The listing builds one solid part. Answer for the finished solid, in the listing's coordinates (mm). A direction names the side the tool comes from. Give positions to 0.01 mm unless a question says otherwise; leave off trailing zeros. One line per question, with ' | ' between items. Start each with the question number.
1. Given P1, Ø17, axis at x = -3.175, y = -38.1, coming from the -Z side; P2, Ø4, axis at x = 17.5, z = -65, coming from the +Y side; P3, Ø15.5, axis at y = 53, z = 56.5, coming from the +X side, each flat-ended and moving along its own axis, determine where each tip first touches the part or whether it passes through.
2. Find the intervals of material crossed by L1, parallel to Y at x = 2, z = 57; L2, parallel to Z at x = -2, y = -23; L3, parallel to X at y = 38.1, z = -165 (3 decimals), in increasing order. Write a range as from..to.
3. The mould has two halves that part along Y. Classify faces 1 (the face through (18, 14.288, 3)), 2 (the face through (22.225, 36, 3)), 3 (the face through (-4, 57.15, 3)): +Y half, -Y half, draft (parallel to the pull), parting line (faces both ways), or undercut.
4. For faces 4 (the face through (-4.415, -47.544, -165.633)), 5 (the face through (18, 28.575, 3)), 6 (the face through (0.31, -22.15, 94.41)), determine the directions among +Z, -Z, +X, -X, +Y, -Y from which every point of the face is accessible in a straight line to the end or side of a thin tool.
5. A cutting plane is placed at B-B (z = -156.5). State how many separate pieces and enclosed holes the cut face has, then the cut area to 3 significant figures.
```python
from build123d import *

# Parameters (mm, degrees)
F1_DEPTH = 203.2
F2_R     = 5.55625
F3_DEPTH = 44.451
F4_R     = 9.525
F5_DEPTH = 76.2


with BuildPart() as f1:
    # F0 (on Top) → F1 (new body, symmetric)
    with BuildSketch(Plane.XY):
        Polygon((14.2875, 57.15), (-22.225, 57.15), (-22.225, -57.15), (22.225, -57.15), (22.225, -42.8625), (14.2875, -42.8625), (14.2875, -28.575), (22.225, -28.575), (22.225, -14.2875), (14.2875, -14.2875), (14.2875, 0), (22.225, 0), (22.225, 14.2875), (14.2875, 14.2875), (14.2875, 28.575), (22.225, 28.575), (22.225, 42.8625), (14.2875, 42.8625), align=None)
    extrude(amount=F1_DEPTH, both=True)

    # F2 (on face) → F3 (cut, through all)
    with BuildSketch(Plane.YZ.offset(22.225)):
        with Locations((-21.43125, 88.9)):
            Circle(F2_R)
        with Locations((-21.43125, 57.15)):
            Circle(F2_R)
    extrude(amount=-F3_DEPTH, mode=Mode.SUBTRACT)

    # F4 (on face) → F5 (cut)
    with BuildSketch(Plane(origin=(0, 0, -203.2), x_dir=(1, 0, 0), z_dir=(0, 0, -1))):
        with Locations((-3.175, -38.1)):
            Circle(F4_R)
        with Locations((-3.175, 38.1)):
            Circle(F4_R)
    extrude(amount=-F5_DEPTH, mode=Mode.SUBTRACT)


solid = f1.part
```
Determined:
1) P1: z = -127 | P2: y = 42.86 | P3: x = 14.29
2) L1: -57.15..-26.99, -15.88..57.15 | L2: -203.2..51.82, 62.48..83.57, 94.23..203.2 | L3: -22.225..-12.7, 6.35..22.225
3) face 1: undercut | face 2: draft | face 3: +Y half
4) face 4: -Z | face 5: +Z, -Z, +X | face 6: +X, -X
5) separate pieces: 1 | enclosed holes: 2 | area: 4,060 mm2
